from build123d import *

# Parameters (mm, degrees)
F1_DEPTH  = 127
F2_W      = 80.2252367139
F2_H      = 66.4800778031
F3_DEPTH  = 127
F4_W      = 17.7462361753
F4_H      = 33.2400389016
F4_W_2    = 16.2856578827
F5_DEPTH  = 152.4
F6_W      = 80.2252367139
F6_H      = 25.0078588724
F7_DEPTH  = 101.6
F8_W      = 27.9699675739
F8_H      = 27.9699731618
F9_DEPTH  = 152.4
F10_DEPTH = 50.8
F11_DEPTH = 106.68
F12_W     = 28.4161847085
F12_H     = 30.0192423165
F13_DEPTH = 96.52
F14_W     = 30.9016443789
F14_H     = 31.186911881
F15_DEPTH = 99.06
F16_W     = 31.6377300769
F16_H     = 35.1597964764
F17_DEPTH = 99.06
F18_R     = 5.08
F19_R     = 5.08


with BuildPart() as f1:
    # F0 (on Front) → F1 (new body)
    with BuildSketch(Plane.XZ):
        Polygon((41.0551093519, 40.1177741587), (-64.293846488, 40.1177741587), (-64.293846488, -37.670340389), (49.9632842839, -37.670340389), (49.9632842839, 40.1177741587), align=None)
    extrude(amount=-F1_DEPTH)

    # F2 (on face) → F3 (cut)
    with BuildSketch(Plane(origin=(0, 127, 0), x_dir=(-1, 0, 0), z_dir=(0, 1, 0))):
        with Locations((7.8955702484, 6.8777352571)):
            Rectangle(F2_W, F2_H)
    extrude(amount=-F3_DEPTH, mode=Mode.SUBTRACT)

    # F4 (on face) → F5 (cut)
    with BuildSketch(Plane(origin=(0, 127, 0), x_dir=(-1, 0, 0), z_dir=(0, 1, 0))):
        with Locations((-41.0901661962, 23.4977547079)):
            Rectangle(F4_W, F4_H)
        with Locations((56.1510175467, 23.4977547079)):
            Rectangle(F4_W_2, F4_H)
    extrude(amount=-F5_DEPTH, mode=Mode.SUBTRACT)

    # F6 (on face) → F7 (join)
    with BuildSketch(Plane.XY.offset(-26.3623036444)):
        with Locations((-7.8955702484, 12.5039294362)):
            Rectangle(F6_W, F6_H)
    extrude(amount=F7_DEPTH)

    # F8 (on face) → F9 (join)
    with BuildSketch(Plane(origin=(0, 0, -37.670340389), x_dir=(1, 0, 0), z_dir=(0, 0, -1))):
        with Locations((-47.3000053316, -17.0427551493)):
            Rectangle(F8_W, F8_H)
    extrude(amount=F9_DEPTH)

    # F10 (add): a face of the model
    f10_faces = [f1.faces().sort_by_distance(p)[0] for p in [
        (-47.3000053316, 17.0427551493, -190.070340389),
    ]]
    extrude(f10_faces, amount=F10_DEPTH)

    # F11 (cut): a face of the model
    f11_faces = [f1.faces().sort_by_distance(p)[0] for p in [
        (-47.3000053316, 17.0427551493, -240.870340389),
    ]]
    extrude(f11_faces, amount=-F11_DEPTH, mode=Mode.SUBTRACT)

    # F12 (on face) → F13 (join)
    with BuildSketch(Plane(origin=(0, 0, -37.670340389), x_dir=(1, 0, 0), z_dir=(0, 0, -1))):
        with Locations((35.7551919296, -15.0096211582)):
            Rectangle(F12_W, F12_H)
    extrude(amount=F13_DEPTH)

    # F14 (on face) → F15 (join)
    with BuildSketch(Plane(origin=(0, 0, -37.670340389), x_dir=(1, 0, 0), z_dir=(0, 0, -1))):
        with Locations((34.5124620944, -111.4065440595)):
            Rectangle(F14_W, F14_H)
    extrude(amount=F15_DEPTH)

    # F16 (on face) → F17 (join)
    with BuildSketch(Plane(origin=(0, 0, -37.670340389), x_dir=(1, 0, 0), z_dir=(0, 0, -1))):
        with Locations((-46.5169167146, -107.4508428574)):
            Rectangle(F16_W, F16_H)
    extrude(amount=F17_DEPTH)

    # F18
    f18_edges = [f1.edges().sort_by_distance(p)[0] for p in [
        (-56.151018, 0, 6.877735),
    ]]
    fillet(f18_edges, radius=F18_R)

    # F19
    f19_edges = [f1.edges().sort_by_distance(p)[0] for p in [
        (41.090166, 0, 6.877735),
    ]]
    fillet(f19_edges, radius=F19_R)


solid = f1.part
Source: CAD feature listing. Evaluate the final solid. Frame: model axes, mm. A direction names the side the tool comes from. Round coordinates to 2 decimals unless told otherwise and drop trailing zeros. Order: outer loops, then holes, each group sorted by start corner. A loop starts at its lowest first (then second) coordinate and runs counter-clockwise, first axis right, second up. Notation, with made-up numbers: (74, -35) - (114, -35) arc R4 cw to (114, -29) - close; hole circle Ø6 at (53.5, 85.5). An arc over 180 degrees is marked (long way). Use a Markdown table: item, result. Add a question column.
1. Section query B-B (y = 118). Return the cut outline in (x, z), then the cut area to 3 significant figures.
2. Section query D-D (z = -5.5). Return the cut outline in (x, y).
3. Section query C-C (x = -18). Return the cut outline in (y, z), then the cut area to 3 significant figures.
4. Mould query, pull axis X, two halves, no side actions, for faces 5 (the flat face through (-61.285, 17, -85)), 6 (the flat face through (19.062, 112, -87)), 7 (the flat face through (32.217, 12, 38)). Classes: +X half, -X half, draft (parallel to the pull), parting line (faces both ways), or undercut.
5. Line query: probe 1 along Y at (x, z) = (-36.5, -47); probe 2 along X at (y, z) = (7.5, -56); probe 3 along Y at (x, z) = (35.5, -62.5). Output: solid intervals per line, ascending.
6. Set-up query: faces 1 (the cylindrical face through (-56, 1.5, 5.4)), 2 (the flat face through (21.547, 15, -85)), 3 (the flat face through (-47, 125.031, -87)), 4 (the flat face through (32.217, 77, -10)). Return all of +Z, -Z, +X, -X, +Y, -Y with unobstructed straight access to the full face (end or side cutting, diameter ignored); none if empty.
7. Section query A-A (z = -49.5). Return the cut outline in (x, y), then the cut area to 3 significant figures.
8. First-contact query: pin 1 (20 mm diameter, centred on y = 13, z = 46.5, fed in from -X); pin 2 (22.5 mm diameter, centred on y = 15, z = -71.5, fed in from -X) (3 decimals); pin 3 (14 mm diameter, centred on x = -54.5, z = -108, fed in from -Y); pin 4 (10 mm diameter, centred on x = 18.5, z = -107.5, fed in from -Y). Flat tips, straight axial feed; report the tip coordinate or a pass-through.
Derived:
| question | item | result |
|---|---|---|
| 1 | outline | (-64.29, -37.67) - (-62.34, -37.67) - (-62.34, -136.73) - (-30.7, -136.73) - (-30.7, -37.67) - (19.06, -37.67) - (19.06, -136.73) - (49.96, -136.73) - (49.96, 6.88) - (32.22, 6.88) - (32.22, -26.36) - (-48.01, -26.36) - (-48.01, 6.88) - (-64.29, 6.88) - close |
| 1 | area | 8,620 mm2 |
| 2 | outline | (-64.29, 0) - (49.96, 0) - (49.96, 127) - (32.22, 127) - (32.22, 25.01) - (-48.01, 25.01) - (-48.01, 127) - (-64.29, 127) - close |
| 3 | outline | (0, -37.67) - (127, -37.67) - (127, -26.36) - (25.01, -26.36) - (25.01, 75.24) - (0, 75.24) - close |
| 3 | area | 3,980 mm2 |
| 4 | face 5 | -X half |
| 4 | face 6 | undercut |
| 4 | face 7 | +X half |
| 5 | probe 1 | 3.06 to 31.03, 89.87 to 125.03 |
| 5 | probe 2 | -61.28 to -33.32, 21.55 to 49.96 |
| 5 | probe 3 | 0 to 30.02, 95.81 to 127 |
| 6 | face 1 | +Z, -X, -Y |
| 6 | face 2 | -Z, -Y |
| 6 | face 3 | -Z, -X, +Y |
| 6 | face 4 | +Z, +Y |
| 7 | outline | (-62.34, 89.87) - (-30.7, 89.87) - (-30.7, 125.03) - (-62.34, 125.03) - close; (-61.28, 3.06) - (-33.32, 3.06) - (-33.32, 31.03) - (-61.28, 31.03) - close; (19.06, 95.81) - (49.96, 95.81) - (49.96, 127) - (19.06, 127) - close; (21.55, 0) - (49.96, 0) - (49.96, 30.02) - (21.55, 30.02) - close |
| 7 | area | 3,710 mm2 |
| 8 | pin 1 | x = -48.01 |
| 8 | pin 2 | x = -61.285 |
| 8 | pin 3 | y = 3.06 |
| 8 | pin 4 | y = 0 |
